from build123d import *

# Parameters (mm, degrees)
BOSS_EXTRUDE2_DEPTH = 2
BOSS_EXTRUDE3_DEPTH = 28.266
SKETCH5_W           = 11.884268041
SKETCH5_H           = 36.556167698
CUT_EXTRUDE3_DEPTH  = 122.459124219
SKETCH7_W           = 8.89
SKETCH7_H           = 3.43
SKETCH7_W_2         = 14.05
SKETCH7_H_2         = 16.84
SKETCH7_W_3         = 17.696
SKETCH7_H_3         = 6.81
SKETCH7_W_4         = 9.3
SKETCH7_H_4         = 11
CUT_EXTRUDE4_DEPTH  = 32


with BuildPart() as part:
    # Sketch1 → Boss-Extrude2 (new body)
    with BuildSketch(Plane.XY):
        with BuildLine():
            Line((-14.4, -41.21), (84, -41.21))
            ThreePointArc((84, -41.21), (85.48492424, -40.59492424), (86.1, -39.11))
            Line((86.1, -39.11), (86.1, 46.79))
            ThreePointArc((86.1, 46.79), (85.48492424, 48.27492424), (84, 48.89))
            Line((84, 48.89), (-14.4, 48.89))
            ThreePointArc((-14.4, 48.89), (-15.88492424, 48.27492424), (-16.5, 46.79))
            Line((-16.5, 46.79), (-16.5, -39.11))
            ThreePointArc((-16.5, -39.11), (-15.88492424, -40.59492424), (-14.4, -41.21))
        make_face()
    extrude(amount=-BOSS_EXTRUDE2_DEPTH)

    # Sketch3 → Boss-Extrude3 (add)
    with BuildSketch(Plane.XY):
        with BuildLine():
            Line((-14.4, -43.21), (84, -43.21))
            ThreePointArc((84, -43.21), (86.899137803, -42.009137803), (88.1, -39.11))
            Line((88.1, -39.11), (88.1, 46.79))
            ThreePointArc((88.1, 46.79), (86.899137803, 49.689137803), (84, 50.89))
            Line((84, 50.89), (-14.4, 50.89))
            ThreePointArc((-14.4, 50.89), (-17.299137803, 49.689137803), (-18.5, 46.79))
            Line((-18.5, 46.79), (-18.5, -39.11))
            ThreePointArc((-18.5, -39.11), (-17.299137803, -42.009137803), (-14.4, -43.21))
        make_face()
    extrude(amount=-BOSS_EXTRUDE3_DEPTH)

    # Sketch5 → Cut-Extrude3 (cut, through all)
    with BuildSketch(Plane(origin=(88.1, 0, 0), x_dir=(0, 0, -1), z_dir=(1, 0, 0))):
        with Locations((8.594465961, 18.278083849)):
            Rectangle(SKETCH5_W, SKETCH5_H)
    extrude(amount=-CUT_EXTRUDE3_DEPTH, mode=Mode.SUBTRACT)

    # Sketch7 → Cut-Extrude4 (cut)
    with BuildSketch(Plane.XZ.offset(43.21)):
        with Locations((76.775, -26.5048)):
            Rectangle(SKETCH7_W, SKETCH7_H)
        Polygon((68.12, -28.296), (69.827, -28.296), (69.827, -14.646007205), (68.12, -14.646007205), (66.12, -14.646007205), (57.38, -14.646007205), (55.38, -14.646007205), (53.673, -14.646007205), (53.673, -28.296), (55.38, -28.296), (57.38, -28.296), (66.12, -28.296), align=None)
        with Locations((44.4, -19.7998)):
            Rectangle(SKETCH7_W_2, SKETCH7_H_2)
        with Locations((27.4, -19.7998)):
            Rectangle(SKETCH7_W_2, SKETCH7_H_2)
        with Locations((7.56, -24.8148)):
            Rectangle(SKETCH7_W_3, SKETCH7_H_3)
        with Locations((-9.2, -22.796)):
            Rectangle(SKETCH7_W_4, SKETCH7_H_4)
    extrude(amount=-CUT_EXTRUDE4_DEPTH, mode=Mode.SUBTRACT)


solid = part.part
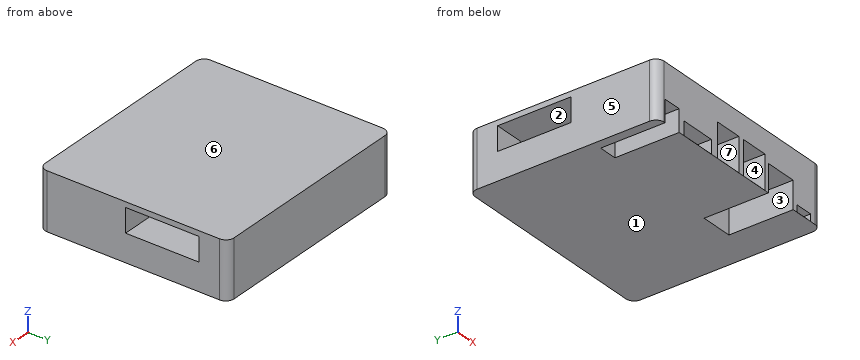
Here's how the part is built. I have some questions about the finished solid (model axes, mm). Face numbers are marked on the shaded views. A direction names the side the tool comes from. Coordinates: 2 decimals unless noted, no trailing zeros. Loops run counter-clockwise (first coordinate to the right, second up) from the corner with the lowest first, then second, coordinate; pieces in that order, holes last. Notation, with made-up numbers: (36.25, -16) -> (52.25, -16) arc R16 cw to (52.25, 9) -> close; hole circle Ø11 at (89, 76). An arc over 180 degrees is marked (long way). Use one line per item in the form item = value. Start each with the question number.
(1) On a 3-axis mill with a long thin cutter (end or side, diameter ignored), from which of +Z, -Z, +X, -X, +Y, -Y can I reach the whole of each face in a straight line? I mean the marked faces 1, 2 and 3. Say none if no direction works.
(2) If we section it at A-A (z = -9.5): Please give me the cut outline in (x, y), then the cut area to 3 significant figures.
(3) We'd pull the mould along X, two halves only. Please class the marked faces 4, 5, 6 and 7: pulls with the +X half, pulls with the -X half, needs draft (parallel to the pull), parting line crosses it, or undercut.
(4) If we section it at D-D (z = -20): Please give me the cut outline in (x, y) (3 decimals), then the cut area to 3 significant figures.
(5) Please list where these lines run through material, in increasing order: line 1 along X through (y, z) = (-29, -13.75) (3 decimals); line 2 along Z through (x, y) = (64.5, 5.5); line 3 along Y through (x, z) = (23.5, -12.25).
(6) Will this pin go through, and if not, where does the flat tip stop? pin 1 (3 mm diameter, centred on x = -10, z = -23.5, fed in from -Y).
(7) If we section it at C-C (x = 74.5): Please give me the cut outline in (y, z), then the cut area to 3 significant figures.
(8) If we section it at B-B (y = 30.5): Please give me the cut outline in (x, z), then the cut area to 3 significant figures.
Verdict:
q1.face_1 = -Z, +X, -X, +Y, -Y
q1.face_2 = +X, -X
q1.face_3 = -Z, -Y
q2.outline = (-18.5, -39.11) arc R4.1 ccw to (-14.4, -43.21) -> (84, -43.21) arc R4.1 ccw to (88.1, -39.11) -> (88.1, 0) -> (-18.5, 0) -> close; (-18.5, 36.56) -> (88.1, 36.56) -> (88.1, 46.79) arc R4.1 ccw to (84, 50.89) -> (-14.4, 50.89) arc R4.1 ccw to (-18.5, 46.79) -> close
q2.area = 6,120 mm²
q3.face_4 = undercut
q3.face_5 = pulls with the -X half
q3.face_6 = needs draft
q3.face_7 = undercut
q4.outline = (-18.5, -39.11) arc R4.1 ccw to (-14.4, -43.21) -> (-13.85, -43.21) -> (-13.85, -11.21) -> (-4.55, -11.21) -> (-4.55, -43.21) -> (20.375, -43.21) -> (20.375, -11.21) -> (34.425, -11.21) -> (34.425, -43.21) -> (37.375, -43.21) -> (37.375, -11.21) -> (51.425, -11.21) -> (51.425, -43.21) -> (53.673, -43.21) -> (53.673, -11.21) -> (69.827, -11.21) -> (69.827, -43.21) -> (84, -43.21) arc R4.1 ccw to (88.1, -39.11) -> (88.1, 46.79) arc R4.1 ccw to (84, 50.89) -> (-14.4, 50.89) arc R4.1 ccw to (-18.5, 46.79) -> close
q4.area = 8,300 mm²
q5.line_1 = -18.5 to 20.375, 34.425 to 37.375, 51.425 to 88.1
q5.line_2 = -28.27 to -14.54, -2.65 to 0
q5.line_3 = -11.21 to 0, 36.56 to 50.89
q6.pin_1 = -11.21
q7.outline = (-43.21, -28.27) -> (50.89, -28.27) -> (50.89, 0) -> (-43.21, 0) -> (-43.21, -24.79) -> (-11.21, -24.79) -> (-11.21, -28.22) -> (-43.21, -28.22) -> close; hole (0, -14.54) -> (36.56, -14.54) -> (36.56, -2.65) -> (0, -2.65) -> close
q7.area = 2,120 mm²
q8.outline = (-18.5, -28.27) -> (88.1, -28.27) -> (88.1, -14.54) -> (-18.5, -14.54) -> close; (-18.5, -2.65) -> (88.1, -2.65) -> (88.1, 0) -> (-18.5, 0) -> close
q8.area = 1,750 mm²
